from build123d import *

# Parameters (mm, degrees)
SKETCH1_W           = 2
SKETCH1_H           = 14
BOSS_EXTRUDE1_DEPTH = 7
SKETCH2_W           = 16
SKETCH2_H           = 16
BOSS_EXTRUDE2_DEPTH = 2
BOSS_EXTRUDE3_DEPTH = 2
BOSS_EXTRUDE4_DEPTH = 2
SKETCH6_W           = 12
SKETCH6_H           = 15
BOSS_EXTRUDE5_DEPTH = 2
SKETCH7_W           = 12
SKETCH7_H           = 16
BOSS_EXTRUDE6_DEPTH = 2
SKETCH8_W           = 12
SKETCH8_H           = 17
BOSS_EXTRUDE7_DEPTH = 2
SKETCH9_W           = 12
SKETCH9_H           = 3.5
BOSS_EXTRUDE9_DEPTH = 1
FILLET1_R           = 3
FILLET2_R           = 10
FILLET3_R           = 2
CUT_EXTRUDE4_REACH  = 32.199
SKETCH14_R          = 1
FILLET4_R           = 2
CUT_EXTRUDE5_DEPTH  = 26.159491251
FILLET5_R           = 2


# Some blends are built 0.0001 mm under size
with BuildPart() as part:
    # Sketch1 → Boss-Extrude1 (new body)
    with BuildSketch(Plane(origin=(0, 0, 0), x_dir=(1, 0, 0), z_dir=(0, 1, 0))):
        with Locations((1, -7)):
            Rectangle(SKETCH1_W, SKETCH1_H)
    extrude(amount=BOSS_EXTRUDE1_DEPTH)

    # Sketch2 → Boss-Extrude2 (add)
    with BuildSketch(Plane(origin=(0, 7, 0), x_dir=(1, 0, 0), z_dir=(0, 1, 0))):
        with Locations((8, -8)):
            Rectangle(SKETCH2_W, SKETCH2_H)
    extrude(amount=BOSS_EXTRUDE2_DEPTH)

    # Sketch4 → Boss-Extrude3 (add)
    with BuildSketch(Plane(origin=(16, 0, 0), x_dir=(0, 0, -1), z_dir=(1, 0, 0))):
        Polygon((0, 0), (15, -11), (15, 9), (0, 9), align=None)
    extrude(amount=-BOSS_EXTRUDE3_DEPTH)

    # Sketch5 → Boss-Extrude4 (add)
    with BuildSketch(Plane.ZY):
        Polygon((0, 9), (-15, 9), (-15, -11), (0, 0), align=None)
    extrude(amount=-BOSS_EXTRUDE4_DEPTH)

    # Sketch6 → Boss-Extrude5 (add)
    with BuildSketch(Plane(origin=(0, 9, 0), x_dir=(1, 0, 0), z_dir=(0, 1, 0))):
        with Locations((8, 7.5)):
            Rectangle(SKETCH6_W, SKETCH6_H)
    extrude(amount=-BOSS_EXTRUDE5_DEPTH)

    # Sketch7 → Boss-Extrude6 (add)
    with BuildSketch(Plane(origin=(0, 0, -15), x_dir=(-1, 0, 0), z_dir=(0, 0, -1))):
        with Locations((-8, -1)):
            Rectangle(SKETCH7_W, SKETCH7_H)
    extrude(amount=-BOSS_EXTRUDE6_DEPTH)

    # Sketch8 → Boss-Extrude7 (add)
    with BuildSketch(Plane(origin=(0, 0, 0), x_dir=(1, 0, 0), z_dir=(0, -0.8064049958557057, 0.5913636636275174))):
        with Locations((8, -8.5)):
            Rectangle(SKETCH8_W, SKETCH8_H)
    extrude(amount=-BOSS_EXTRUDE7_DEPTH)

    # Sketch9 → Boss-Extrude9 (add)
    with BuildSketch(Plane.XZ):
        with Locations((8, -0.25)):
            Rectangle(SKETCH9_W, SKETCH9_H)
    extrude(amount=-BOSS_EXTRUDE9_DEPTH)

    # Fillet1
    fillet1_edges = [part.edges().sort_by_distance(p)[0] for p in [
        (8, 9, -15),
    ]]
    fillet(fillet1_edges, radius=FILLET1_R)

    # Fillet2
    # the kernel refuses this fillet: 10 mm, written as the material it adds along each edge
    with BuildSketch(Plane(origin=(0, 0, 0), x_dir=(0, -0.5913636636275174, -0.8064049958557056), z_dir=(1, 0, 0))) as fillet2_piece_1_section:
        with BuildLine():
            CenterArc((FILLET2_R * 0.327370476158, -FILLET2_R), FILLET2_R, 90, 36.253837737)
            Line((-FILLET2_R * 0.263993187469, -FILLET2_R * 0.193595004144), (0, 0))
            Line((0, 0), (FILLET2_R * 0.327370476158, 0))
        make_face()
    fillet2_piece_1 = extrude(amount=14, mode=Mode.PRIVATE)
    fillet2_piece_1 = split(fillet2_piece_1, bisect_by=Plane(origin=(1, -0.664008542, 1.5), z_dir=(0, 0, -1)), keep=Keep.TOP, mode=Mode.PRIVATE)
    add(fillet2_piece_1)
    with BuildSketch(Plane(origin=(0, 0, 0), x_dir=(0, -0.5913636636275174, -0.8064049958557056), z_dir=(1, 0, 0))) as fillet2_piece_2_section:
        with BuildLine():
            CenterArc((FILLET2_R * 0.327370476158, -FILLET2_R), FILLET2_R, 90, 36.253837737)
            Line((-FILLET2_R * 0.263993187469, -FILLET2_R * 0.193595004144), (0, 0))
            Line((0, 0), (FILLET2_R * 0.327370476158, 0))
        make_face()
    fillet2_piece_2 = extrude(amount=22.184261904, mode=Mode.PRIVATE)
    fillet2_piece_2 = split(fillet2_piece_2, bisect_by=Plane(origin=(2, -0.047502187, 1.942720069), z_dir=(-1, 0, 0)), keep=Keep.TOP, mode=Mode.PRIVATE)
    add(fillet2_piece_2)

    # Fillet3
    fillet3_edges = [part.edges().sort_by_distance(p)[0] for p in [
        (8, 9, 16),
    ]]
    fillet(fillet3_edges, radius=FILLET3_R - 0.0001)  # a hair under: the kernel refuses the full size

    # Sketch14 → Cut-Extrude4 (cut, up to next)
    with BuildSketch(Plane(origin=(0, 9, 0), x_dir=(1, 0, 0), z_dir=(0, 1, 0)), mode=Mode.PRIVATE) as cut_extrude4_sk1:
        with Locations(Location((4, -12, 0), (0, 0, 270))):
            Circle(SKETCH14_R)
    cut_extrude4_tool1 = extrude(cut_extrude4_sk1.sketch, amount=-CUT_EXTRUDE4_REACH, mode=Mode.PRIVATE) & part.part
    # Sketch14 → Cut-Extrude4 (cut, up to next)
    with BuildSketch(Plane(origin=(0, 9, 0), x_dir=(1, 0, 0), z_dir=(0, 1, 0)), mode=Mode.PRIVATE) as cut_extrude4_sk2:
        with Locations(Location((4, -4, 0), (0, 0, 270))):
            Circle(SKETCH14_R)
    cut_extrude4_tool2 = extrude(cut_extrude4_sk2.sketch, amount=-CUT_EXTRUDE4_REACH, mode=Mode.PRIVATE) & part.part
    # Sketch14 → Cut-Extrude4 (cut, up to next)
    with BuildSketch(Plane(origin=(0, 9, 0), x_dir=(1, 0, 0), z_dir=(0, 1, 0)), mode=Mode.PRIVATE) as cut_extrude4_sk3:
        with Locations(Location((12, -12, 0), (0, 0, 270))):
            Circle(SKETCH14_R)
    cut_extrude4_tool3 = extrude(cut_extrude4_sk3.sketch, amount=-CUT_EXTRUDE4_REACH, mode=Mode.PRIVATE) & part.part
    # Sketch14 → Cut-Extrude4 (cut, up to next)
    with BuildSketch(Plane(origin=(0, 9, 0), x_dir=(1, 0, 0), z_dir=(0, 1, 0)), mode=Mode.PRIVATE) as cut_extrude4_sk4:
        with Locations(Location((12, -4, 0), (0, 0, 270))):
            Circle(SKETCH14_R)
    cut_extrude4_tool4 = extrude(cut_extrude4_sk4.sketch, amount=-CUT_EXTRUDE4_REACH, mode=Mode.PRIVATE) & part.part
    add(cut_extrude4_tool1.solids().sort_by_distance((4, 9, 12))[0], mode=Mode.SUBTRACT)
    add(cut_extrude4_tool2.solids().sort_by_distance((4, 9, 4))[0], mode=Mode.SUBTRACT)
    add(cut_extrude4_tool3.solids().sort_by_distance((12, 9, 12))[0], mode=Mode.SUBTRACT)
    add(cut_extrude4_tool4.solids().sort_by_distance((12, 9, 4))[0], mode=Mode.SUBTRACT)

    # Fillet4
    # the kernel refuses this fillet: 2 mm, written as the material it takes off along each edge
    with BuildSketch(Plane(origin=(14, 1.612809992, -1.182727327), x_dir=(0, -0.5913636636275179, -0.806404995855705), z_dir=(-1, 0, 0))) as fillet4_piece_1:
        with BuildLine():
            CenterArc((1.569146973, 2), FILLET4_R, 218.318751839, 51.681248161)
            Line((0, 0.759928317), (-0.031382939, 0.735126884))
            ThreePointArc((-0.031382939, 0.735126884), (-0.04, 0.379964159), (-0.04, 0))
            Line((-0.04, 0), (0, -0.04))
            Line((0, -0.04), (1.569146973, -0.04))
            Line((1.569146973, -0.04), (1.569146973, 0))
        make_face()
    extrude(amount=12, mode=Mode.SUBTRACT)

    # Sketch15 → Cut-Extrude5 (cut, through all)
    with BuildSketch(Plane(origin=(16, 0, 0), x_dir=(0, 0, -1), z_dir=(1, 0, 0))):
        Polygon((13.636363636, -10), (15, -11), (15, -9), align=None)
    extrude(amount=-CUT_EXTRUDE5_DEPTH, mode=Mode.SUBTRACT)

    # Fillet5
    # the kernel refuses this fillet: 2 mm, written as the material it takes off along each edge
    with BuildSketch(Plane(origin=(19.666666667, -10, -13.636363636), x_dir=(0, 0.5913636636275166, 0.806404995855706), z_dir=(-1, 0, 0))) as fillet5_piece_1:
        with BuildLine():
            CenterArc((FILLET5_R * 0.733333333333, FILLET5_R), FILLET5_R, 197.492324525, 72.507675475)
            Line((-FILLET5_R * 0.2204238921, FILLET5_R * 0.699421965318), (0, 0))
            Line((0, 0), (FILLET5_R * 0.733333333333, 0))
        make_face()
    extrude(amount=23.333333333, mode=Mode.SUBTRACT)


solid = part.part
Read the model definition and answer for the solid it produces. Units are mm, in the model's axes. A direction names the side the tool comes from. Round coordinates to 2 decimals unless told otherwise and drop trailing zeros. Order: outer loops, then holes, each group sorted by start corner. A loop starts at its lowest first (then second) coordinate and runs counter-clockwise, first axis right, second up.
1) For faces 1 (the face through (4.676, 8.014, 11.263)), 2 (the face through (8, 7, 1)), 3 (the face through (2, 3, -2)), 4 (the face through (15, 4, 0)), determine the directions among +Z, -Z, +X, -X, +Y, -Y from which every point of the face is accessible in a straight line to the end or side of a thin tool.
2) The part is cut by section A-A on x = 12. Give the number of separate pieces and of enclosed holes in the cut face, plus the area to 3 significant figures.
3) The part is cut by section B-B on z = 4. Write down the section's boundary in (x, y), plus the area to 3 significant figures.
4) Flat-ended cylindrical pins translate along their axes: pin 1 (1 mm diameter, centred on y = 5, z = -5, fed in from -X); pin 2 (6 mm diameter, centred on x = 8, z = -5, fed in from -Y); pin 3 (1.6 mm diameter, centred on x = 14.5, y = 2.5, fed in from +Z); pin 4 (1.3 mm diameter, centred on x = 8.5, y = 0.5, fed in from +Z). Find the tip coordinate at first contact, or state that the pin passes through.
5) The part is cut by section D-D on y = -3. Write down the section's boundary in (x, z), plus the area to 3 significant figures.
6) Straight lines are drawn through the part: L1, parallel to X at y = 8.2, z = 12; L2, parallel to X at y = 5.5, z = -9; L3, parallel to X at y = 1.5, z = 4. For each, find the intervals that lie inside material, in ascending order.
7) The mould has two halves that part along Y. Classify faces 5 (the face through (14, 0.1, 0.4)), 6 (the face through (8.084, 1.041, -1.614)), 7 (the face through (1, 0, 9)), 8 (the face through (8, 1, 0)): released by +Y, released by -Y, zero draft, split by the parting line, or undercut.
Resolved:
1. face 1: +Y, -Y
1. face 2: +Z
1. face 3: none
1. face 4: +Z, +X, -Y
2. separate pieces: 3
2. enclosed holes: 0
2. area: 117 mm2
3. outline: (0, 0) - (2, 0) - (2, 7) - (3, 7) - (3, 9) - (0, 9) - close; (5, 7) - (11, 7) - (11, 9) - (5, 9) - close; (13, 7) - (16, 7) - (16, 9) - (13, 9) - close
3. area: 38.0 mm2
4. pin 1: stops at x = 0
4. pin 2: stops at y = -5.87
4. pin 3: stops at z = 0
4. pin 4: stops at z = 1.5
5. outline: (0, -15) - (16, -15) - (16, -4.09) - (0, -4.09) - close; hole (2, -13) - (14, -13) - (14, -7.47) - (2, -7.47) - close
5. area: 108 mm2
6. L1: x = 0 to 3, 5 to 11, 13 to 16
6. L2: x = 0 to 2, 14 to 16
6. L3: x = 0 to 2
7. face 5: zero draft
7. face 6: undercut
7. face 7: released by -Y
7. face 8: undercut
